Source: three-view drawing plus pictorial views. Frame: mm from the lowest corner of the part. A direction names the side the tool comes from. Coordinates: 2 decimals unless noted, no trailing zeros. Order: outer loops, then holes, each group sorted by start corner. A loop starts at its lowest first (then second) coordinate and runs counter-clockwise, first axis right, second up. Notation, with made-up numbers: (6.25, 67) - (34.25, 67) arc R9 ccw to (34.25, 73) - close; hole circle Ø10 at (8.25, 41.25). An arc over 180 degrees is marked (long way). One line per question, with ' | ' between items.
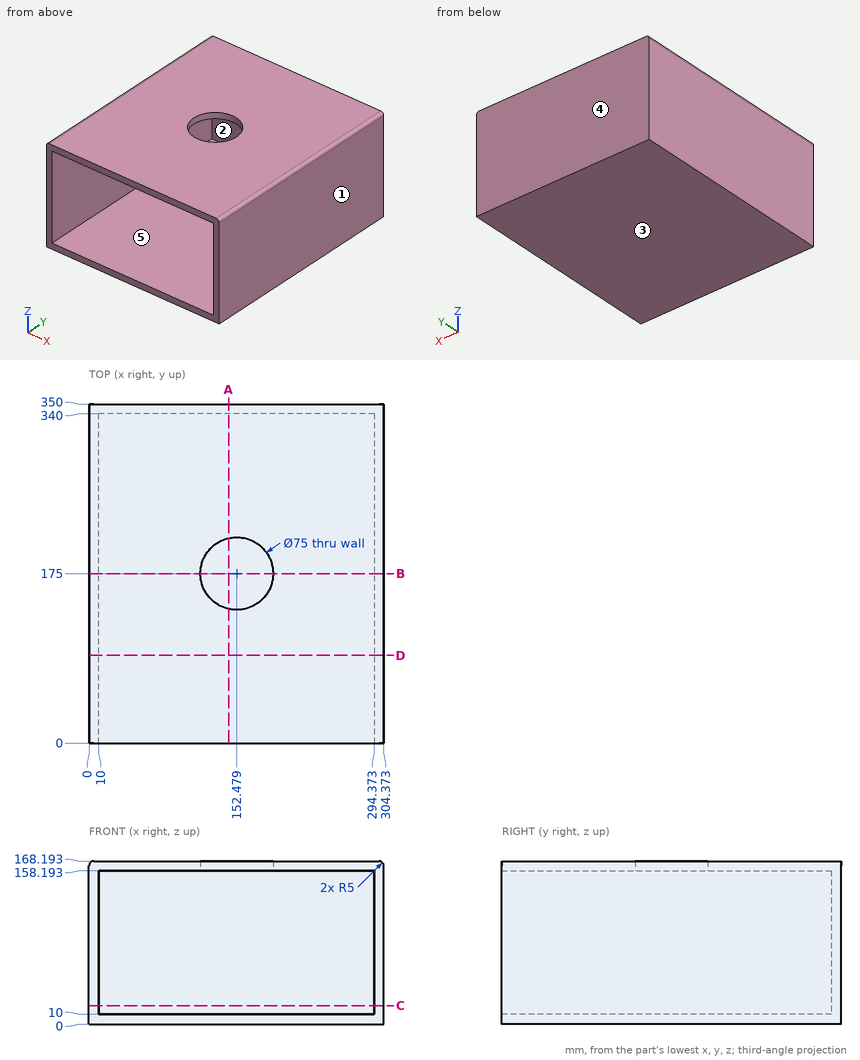
(1) Material intervals for L1, parallel to Z at x = 15, y = 141; L2, parallel to X at y = 61.5, z = 87; L3, parallel to Y at x = 65.5, z = 111.5, sorted ascending. Write a range as from..to.
Taken from the geometry:
L1: z = 0..10, 158.19..168.19 | L2: x = 0..10, 294.37..304.37 | L3: y = 340..350
(2) Pull-direction query (Z, two-part tool) for the marked faces 3, 4 and 5; classes: pulls with the +Z half, pulls with the -Z half, needs draft (parallel to the pull), parting line crosses it, or undercut.
Taken from the geometry:
face 3: pulls with the -Z half | face 4: needs draft | face 5: undercut
(3) Cut plane B-B (y = 175). Return the cut outline in (x, z).
Taken from the geometry:
outline: (0, 0) - (304.37, 0) - (304.37, 163.19) arc R5 ccw to (299.37, 168.19) - (189.98, 168.19) - (189.98, 158.19) - (294.37, 158.19) - (294.37, 10) - (10, 10) - (10, 158.19) - (114.98, 158.19) - (114.98, 168.19) - (5, 168.19) arc R5 ccw to (0, 163.19) - close
(4) Cut plane C-C (z = 19). Return the cut outline in (x, y).
Taken from the geometry:
outline: (0, 0) - (10, 0) - (10, 340) - (294.37, 340) - (294.37, 0) - (304.37, 0) - (304.37, 350) - (0, 350) - close
(5) Pin query (flat end, axial travel): P1, Ø12, axis at x = 173, y = 194.5, coming from the +Z side; P2, Ø2, axis at x = 169, z = 82.5, coming from the -Y side; P3, Ø8, axis at y = 159.5, z = 149, coming from the -X side. Return the tip coordinate at first contact, or that it passes through.
Taken from the geometry:
P1: stops at z = 10 | P2: stops at y = 340 | P3: stops at x = 0
(6) Cut plane D-D (y = 90.5). Return the cut outline in (x, z).
Taken from the geometry:
outline: (0, 0) - (304.37, 0) - (304.37, 163.19) arc R5 ccw to (299.37, 168.19) - (5, 168.19) arc R5 ccw to (0, 163.19) - close; hole (10, 10) - (294.37, 10) - (294.37, 158.19) - (10, 158.19) - close
(7) Set-up query: the marked faces 1 and 2. Return all of +Z, -Z, +X, -X, +Y, -Y with unobstructed straight access to the full face (end or side cutting, diameter ignored); none if empty.
Taken from the geometry:
face 1: +Z, -Z, +X, +Y, -Y | face 2: -Y
(8) Cut plane A-A (x = 144). Return the cut outline in (y, z).
Taken from the geometry:
outline: (0, 0) - (350, 0) - (350, 168.19) - (211.53, 168.19) - (211.53, 158.19) - (340, 158.19) - (340, 10) - (0, 10) - close; (0, 158.19) - (138.47, 158.19) - (138.47, 168.19) - (0, 168.19) - close
